The model under review builds one solid part; all positions refer to its coordinate system, in mm. Face numbers are marked on the shaded views. A direction names the side the tool comes from. Coordinates: 2 decimals unless noted, no trailing zeros. Order: outer loops, then holes, each group sorted by start corner. A loop starts at its lowest first (then second) coordinate and runs counter-clockwise, first axis right, second up. Notation, with made-up numbers: M -23.75,50.5 L -3.75,50.5 A22 cw -3.75,65.5 Z; hole C 39,-36.75 d10. An arc over 180 degrees is marked long. Answer in a Markdown table with one row per item.
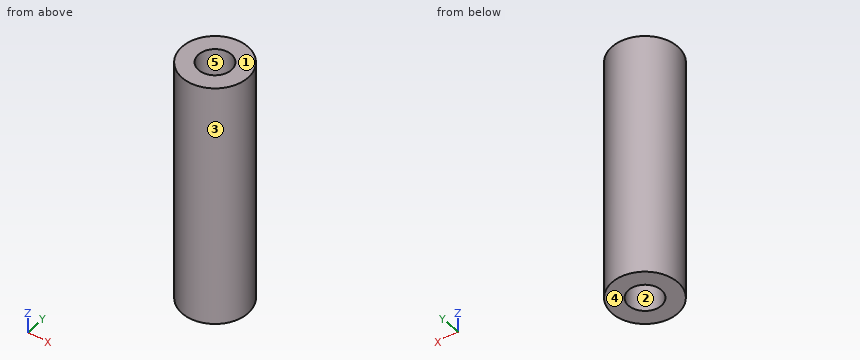
Autodesk Inventor part; units mm, degrees
ref_plane "YZ Plane" through (0, 0, 0) normal (1, 0, 0) x (0, 1, 0)
ref_plane "XZ Plane" through (0, 0, 0) normal (0, 1, 0) x (-1, 0, 0)
ref_plane "XY Plane" through (0, 0, 0) normal (0, 0, 1) x (1, 0, 0)
sketch "スケッチ1" plane through (0, 0, 0) normal (0, 0, 1) x (1, 0, 0)
  circle A0 centre (0, 0) radius 4
  dimension "d0" = 8
extrude "押し出し1" add sketch "スケッチ1" along normal blind 30
hole "穴1" at (0, 0, 0) direction (0, 0, 1) diameter 4 depth 8 tip angle 118
sketch "スケッチ2" plane through (0, 0, 30) normal (0, 0, 1) x (1, 0, 0)
  point P0 (0, 0)
  point P1 (0, 0)
hole "穴2" at (0, 0, 30) direction (0, 0, -1) diameter 4 depth 8 tip angle 118
properties part number "スペーサ　m4-l30" material "アルミニウム 2014-T4"
(1) To check wall thickness, follow line 1 (Y direction, x = 0, z = 24.5); line 2 (Y direction, x = 1, z = 21.75); line 3 (X direction, y = 1.75, z = 24). State the ranges of each line that lie inside material, in increasing order. Write a range as [from, to].
Report:
| item | result |
|---|---|
| line 1 | [-4, -2], [2, 4] |
| line 2 | [-3.87, -1.23], [1.23, 3.87] |
| line 3 | [-3.6, -0.97], [0.97, 3.6] |
(2) Take a section at B-B (z = 17.25). Write out the cut boundary in (x, y), then the cut area to 3 significant figures.
Report:
| item | result |
|---|---|
| outline | C 0,0 d8 |
| area | 50.3 mm^2 |
(3) Machinability: for the marked faces 1 and 2, which of the approach directions +Z, -Z, +X, -X, +Y, -Y give a long, thin tool a straight path to every point of the face, cutting with its end or side? Answer none if there is none.
Report:
| item | result |
|---|---|
| face 1 | +Z, +X, -X, +Y, -Y |
| face 2 | -Z |
(4) Insertion check: P1, Ø3, axis at x = 0, y = 0, coming from the -Z side; P2, Ø1.5, axis at x = -0.5, z = 10, coming from the -Y side. Each pin has a flat end and moves straight along its axis. Give the tip position at first contact, or say it passes through.
Report:
| item | result |
|---|---|
| P1 | z = 8.3 |
| P2 | y = -4 |
(5) The part is to be moulded in two halves that separate along Y. For the marked faces 3, 4 and 5, say which applies: +Y half, -Y half, draft (parallel to the pull), parting line (faces both ways), or undercut.
Report:
| item | result |
|---|---|
| face 3 | parting line |
| face 4 | draft |
| face 5 | undercut |
(6) Take a section at A-A (z = 7.25). Write out the cut boundary in (x, y), then the cut area to 3 significant figures.
Report:
| item | result |
|---|---|
| outline | C 0,0 d8; hole C 0,0 d4 |
| area | 37.7 mm^2 |
(7) Take a section at C-C (x = -2.75). Write out the cut boundary in (y, z).
Report:
| item | result |
|---|---|
| outline | M -2.9,0 L 2.9,0 L 2.9,30 L -2.9,30 Z |
(8) Take a section at D-D (y = 3.25). Write out the cut boundary in (x, z).
Report:
| item | result |
|---|---|
| outline | M -2.33,0 L 2.33,0 L 2.33,30 L -2.33,30 Z |
